Read the model definition and answer for the solid it produces. Units are mm, in the model's axes. Face numbers are marked on the shaded views. A direction names the side the tool comes from. Round coordinates to 2 decimals unless told otherwise and drop trailing zeros. Loops run counter-clockwise (first coordinate to the right, second up) from the corner with the lowest first, then second, coordinate; pieces in that order, holes last. Notation, with made-up numbers: (43.25, -3.5) - (67.25, -3.5) arc R26 cw to (67.25, 24.5) - close; hole circle Ø10 at (67.5, 65.5). An arc over 180 degrees is marked (long way). Answer as CSV lines item,"result".
```python
from build123d import *

# Parameters (mm, degrees)
F0_R     = 16.548871
F1_DEPTH = 5
F2_R     = 11.611904
F3_DEPTH = 5
F4_W     = 5.000622
F4_H     = 32.099514
F5_DEPTH = 5


with BuildPart() as f1:
    # F0 (on Top) → F1 (new body)
    with BuildSketch(Plane.XY):
        Circle(F0_R)
    extrude(amount=F1_DEPTH)

    # F2 (on face) → F3 (cut)
    with BuildSketch(Plane.XY.offset(5)):
        Circle(F2_R)
    extrude(amount=-F3_DEPTH, mode=Mode.SUBTRACT)

    # F4 (on Top) → F5 (join)
    with BuildSketch(Plane.XY):
        with Locations((16.688134, -0.253783)):
            Rectangle(F4_W, F4_H)
    extrude(amount=F5_DEPTH)


solid = f1.part
```
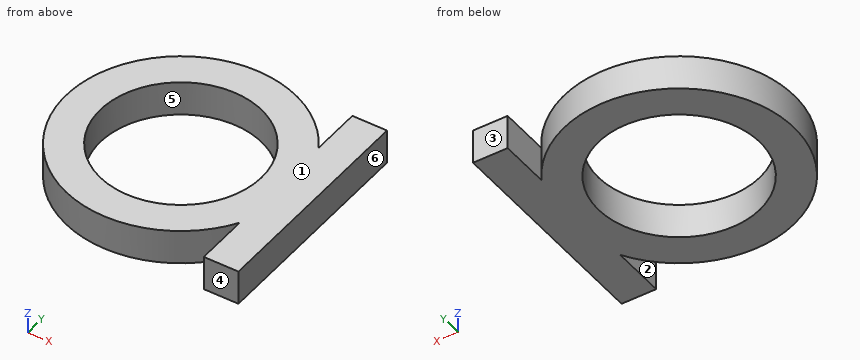
1) A tool of negligible diameter and unlimited length cuts with its end or side. For the marked faces 1 and 2, from which of +Z, -Z, +X, -X, +Y, -Y can it reach the whole face along a straight path? Write none if from no direction.
Entries:
face 1,"+Z, +X, -X, +Y, -Y"
face 2,"+Z, -Z, -Y"
2) A cutting plane is placed at B-B, the plane y = -14. Determine the outline of the cut face in (x, z), plus the area to 3 significant figures.
Entries:
outline,"(-8.82, 0) - (8.82, 0) - (8.82, 5) - (-8.82, 5) - close; (14.19, 0) - (19.19, 0) - (19.19, 5) - (14.19, 5) - close"
area,"113 mm^2"
3) Each of these flat-tipped pins is pushed along its axis until it touches: P1, Ø1.5, axis at x = 15.5, z = 1.5, coming from the +Y side; P2, Ø3, axis at y = -4.5, z = 2, coming from the -X side; P3, Ø1.5, axis at x = 17.5, z = 3, coming from the -Y side; P4, Ø5, axis at x = 8, y = 0, coming from the +Z side. Where does it stop, or does it pass through?
Entries:
P1,"stops at y = 15.8"
P2,"stops at x = -16.27"
P3,"stops at y = -16.3"
P4,"passes through"
4) A cutting plane is placed at D-D, the plane y = -9. Determine the outline of the cut face in (x, z), plus the area to 3 significant figures.
Entries:
outline,"(-13.89, 0) - (-7.34, 0) - (-7.34, 5) - (-13.89, 5) - close; (7.34, 0) - (13.89, 0) - (13.89, 5) - (7.34, 5) - close; (14.19, 0) - (19.19, 0) - (19.19, 5) - (14.19, 5) - close"
area,"90.5 mm^2"
5) A cutting plane is placed at C-C, the plane z = 3.8. Determine the outline of the cut face in (x, y).
Entries:
outline,"(14.19, -16.3) - (19.19, -16.3) - (19.19, 15.8) - (14.19, 15.8) - (14.19, 8.52) arc R16.55 ccw (long way) to (14.19, -8.52) - close; hole circle Ø23.22 at (0, 0)"
6) A cutting plane is placed at A-A, the plane x = 0. Determine the outline of the cut face in (y, z).
Entries:
outline,"(-16.55, 0) - (-11.61, 0) - (-11.61, 5) - (-16.55, 5) - close; (11.61, 0) - (16.55, 0) - (16.55, 5) - (11.61, 5) - close"
7) Find the intervals of material crossed by line 1 (Y direction, x = 0, z = 3.6); line 2 (X direction, y = 14, z = 2.9); line 3 (Y direction, x = 5.5, z = 2.5), in increasing order.
Entries:
line 1,"y = -16.55 to -11.61, 11.61 to 16.55"
line 2,"x = -8.82 to 8.82, 14.19 to 19.19"
line 3,"y = -15.61 to -10.23, 10.23 to 15.61"
8) The mould has two halves that part along Y. Classify the marked faces 3, 4, 5 and 6: pulls with the +Y half, pulls with the -Y half, needs draft (parallel to the pull), parting line crosses it, or undercut.
Entries:
face 3,"pulls with the +Y half"
face 4,"pulls with the -Y half"
face 5,"undercut"
face 6,"needs draft"
